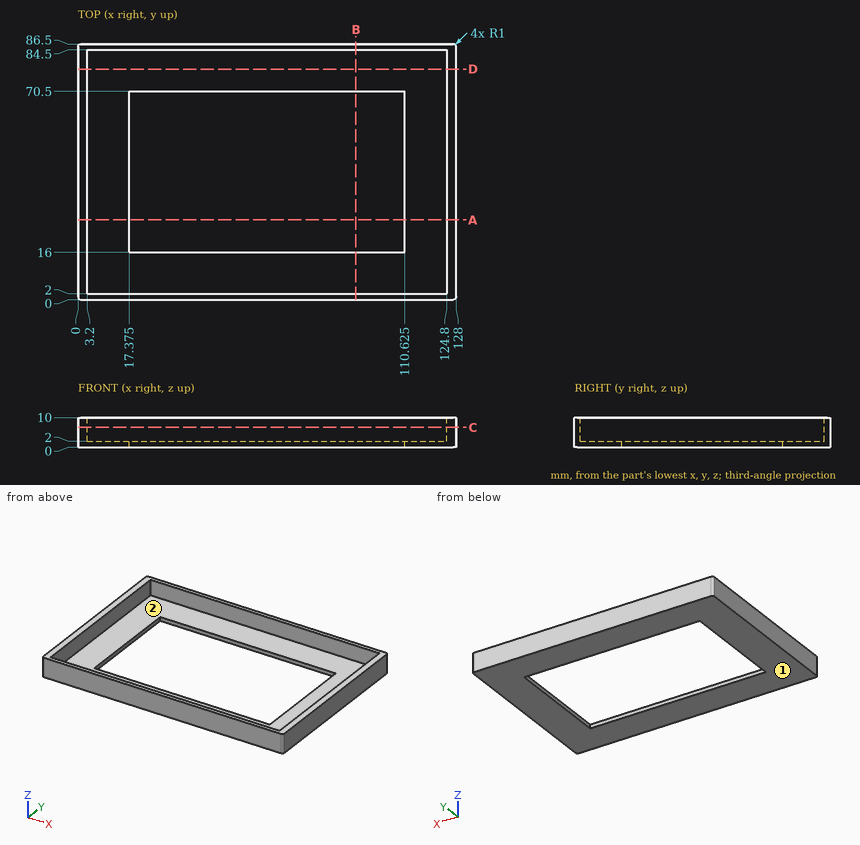
Check sheet for the drawn part. Datum: minimum x, y, z corner. Units: mm. Give positions to 0.01 mm unless a question says otherwise; leave off trailing zeros. Order: outer loops, then holes, each group sorted by start corner. A loop starts at its lowest first (then second) coordinate and runs counter-clockwise, first axis right, second up.
1. Sectioned sample at B-B (x = 94). Record the boundary of the cut face in (y, z).
Completed:
outline: (0, 0) - (16, 0) - (16, 2) - (2, 2) - (2, 10) - (0, 10) - close; (70.5, 0) - (86.5, 0) - (86.5, 10) - (84.5, 10) - (84.5, 2) - (70.5, 2) - close
2. Sectioned sample at A-A (y = 27). Record the boundary of the cut face in (x, z) (3 decimals).
Completed:
outline: (0, 0) - (17.375, 0) - (17.375, 2) - (3.2, 2) - (3.2, 10) - (0, 10) - close; (110.625, 0) - (128, 0) - (128, 10) - (124.8, 10) - (124.8, 2) - (110.625, 2) - close
3. Scan lines: line 1 (X direction, y = 65, z = 6); line 2 (Y direction, x = 78.5, z = 8.5); line 3 (Y direction, x = 104, z = 0.5). Record each from-to range of solid material in increasing order.
Completed:
line 1: x = 0 to 3.2, 124.8 to 128
line 2: y = 0 to 2, 84.5 to 86.5
line 3: y = 0 to 16, 70.5 to 86.5
4. Draft check along X on the marked faces 1 and 2. Enter one of: pulls with the +X half, pulls with the -X half, needs draft (parallel to the pull), parting line crosses it, or undercut.
Completed:
face 1: needs draft
face 2: undercut
5. Sectioned sample at C-C (z = 6.75). Record the boundary of the cut face in (x, y).
Completed:
outline: (0, 1) arc R1 ccw to (1, 0) - (127, 0) arc R1 ccw to (128, 1) - (128, 85.5) arc R1 ccw to (127, 86.5) - (1, 86.5) arc R1 ccw to (0, 85.5) - close; hole (3.2, 2) - (124.8, 2) - (124.8, 84.5) - (3.2, 84.5) - close
6. Depth check by flat-ended pin: pin 1 (10 mm diameter, centred on x = 73, y = 17.5, fed in from +Z). Enter the tip coordinate at first touch or a pass-through.
Completed:
pin 1: stops at z = 2
7. Sectioned sample at D-D (y = 78). Record the boundary of the cut face in (x, z), then the cut area to 3 significant figures.
Completed:
outline: (0, 0) - (128, 0) - (128, 10) - (124.8, 10) - (124.8, 2) - (3.2, 2) - (3.2, 10) - (0, 10) - close
area: 307 mm2
